For this review, take the finished solid that the model builds, in its own axes (mm). A direction names the side the tool comes from. Round coordinates to 2 decimals unless told otherwise and drop trailing zeros. Write each loop counter-clockwise with the first axis right and the second up, starting at its lowest first coordinate (ties: lowest second). Pieces come first, ordered by that corner, then holes. Notation, with made-up numbers: (54, 35.5) -> (71, 35.5) arc R14 ccw to (71, 59.5) -> close; hole circle Ø1 at (53.5, 36.25). An arc over 180 degrees is marked (long way). Answer in a Markdown table with one row per item. Add a question column.
```python
from build123d import *

# Parameters (mm, degrees)
SKETCH1_R           = 1.75
SKETCH1_W           = 15
SKETCH1_H           = 5.2
SKETCH1_W_2         = 5.2
SKETCH1_H_2         = 30
SKETCH1_H_3         = 15
BOSS_EXTRUDE1_DEPTH = 5


with BuildPart() as part:
    # Sketch1 → Boss-Extrude1 (new body)
    with BuildSketch(Plane(origin=(0, 0, 0), x_dir=(1, 0, 0), z_dir=(0, 1, 0))):
        Polygon((92.514530464, -147.019914311), (92.514530464, 52.980085689), (-80.485469536, 52.980085689), (-130.485469536, 27.980085689), (-213.485469536, 27.980085689), (-213.485469536, -122.019914311), (-130.485469536, -122.019914311), (-80.485469536, -147.019914311), align=None)
        with Locations(Location((62.864530464, -134.489914311, 0), (0, 0, 270))):
            Circle(SKETCH1_R, mode=Mode.SUBTRACT)
        with Locations(Location((41.164530464, -134.489914311, 0), (0, 0, 270))):
            Circle(SKETCH1_R, mode=Mode.SUBTRACT)
        with Locations(Location((62.864530464, -128.139914311, 0), (0, 0, 270))):
            Circle(SKETCH1_R, mode=Mode.SUBTRACT)
        with Locations(Location((41.164530464, -128.139914311, 0), (0, 0, 270))):
            Circle(SKETCH1_R, mode=Mode.SUBTRACT)
        with Locations(Location((62.864530464, -115.439914311, 0), (0, 0, 270))):
            Circle(SKETCH1_R, mode=Mode.SUBTRACT)
        with Locations(Location((41.164530464, -115.439914311, 0), (0, 0, 270))):
            Circle(SKETCH1_R, mode=Mode.SUBTRACT)
        with Locations(Location((62.864530464, -102.739914311, 0), (0, 0, 270))):
            Circle(SKETCH1_R, mode=Mode.SUBTRACT)
        with Locations(Location((41.164530464, -102.739914311, 0), (0, 0, 270))):
            Circle(SKETCH1_R, mode=Mode.SUBTRACT)
        with Locations(Location((41.164530464, 8.700085689, 0), (0, 0, 90))):
            Circle(SKETCH1_R, mode=Mode.SUBTRACT)
        with Locations(Location((41.164530464, 21.400085689, 0), (0, 0, 90))):
            Circle(SKETCH1_R, mode=Mode.SUBTRACT)
        with Locations(Location((41.164530464, 34.100085689, 0), (0, 0, 90))):
            Circle(SKETCH1_R, mode=Mode.SUBTRACT)
        with Locations(Location((41.164530464, 40.450085689, 0), (0, 0, 90))):
            Circle(SKETCH1_R, mode=Mode.SUBTRACT)
        with Locations(Location((62.864530464, 8.700085689, 0), (0, 0, 90))):
            Circle(SKETCH1_R, mode=Mode.SUBTRACT)
        with Locations(Location((62.864530464, 21.400085689, 0), (0, 0, 90))):
            Circle(SKETCH1_R, mode=Mode.SUBTRACT)
        with Locations(Location((62.864530464, 34.100085689, 0), (0, 0, 90))):
            Circle(SKETCH1_R, mode=Mode.SUBTRACT)
        with Locations(Location((62.864530464, 40.450085689, 0), (0, 0, 90))):
            Circle(SKETCH1_R, mode=Mode.SUBTRACT)
        with Locations((75.014530464, 47.380085689)):
            Rectangle(SKETCH1_W, SKETCH1_H, mode=Mode.SUBTRACT)
        with Locations((75.014530464, -141.419914311)):
            Rectangle(SKETCH1_W, SKETCH1_H, mode=Mode.SUBTRACT)
        with Locations((86.914530464, -0.019914311)):
            Rectangle(SKETCH1_W_2, SKETCH1_H_2, mode=Mode.SUBTRACT)
        with Locations((86.914530464, -47.019914311)):
            Rectangle(SKETCH1_W_2, SKETCH1_H_2, mode=Mode.SUBTRACT)
        with Locations((86.914530464, -94.019914311)):
            Rectangle(SKETCH1_W_2, SKETCH1_H_2, mode=Mode.SUBTRACT)
        with Locations((-9.785469536, 47.373767599)):
            Rectangle(SKETCH1_W, SKETCH1_H, mode=Mode.SUBTRACT)
        with Locations((-47.985469536, 47.373767599)):
            Rectangle(SKETCH1_W, SKETCH1_H, mode=Mode.SUBTRACT)
        with Locations((-148.485469536, 22.380085689)):
            Rectangle(SKETCH1_W, SKETCH1_H, mode=Mode.SUBTRACT)
        with Locations((-190.985469536, 22.380085689)):
            Rectangle(SKETCH1_W, SKETCH1_H, mode=Mode.SUBTRACT)
        with Locations((-207.885469536, -3.519914311)):
            Rectangle(SKETCH1_W_2, SKETCH1_H_3, mode=Mode.SUBTRACT)
        with Locations((-207.885469536, -47.019914311)):
            Rectangle(SKETCH1_W_2, SKETCH1_H_2, mode=Mode.SUBTRACT)
        with Locations((-207.885469536, -90.519914311)):
            Rectangle(SKETCH1_W_2, SKETCH1_H_3, mode=Mode.SUBTRACT)
        with Locations((-48.86060515, -141.420106162)):
            Rectangle(SKETCH1_W, SKETCH1_H, mode=Mode.SUBTRACT)
        with Locations((-148.485469536, -116.419914311)):
            Rectangle(SKETCH1_W, SKETCH1_H, mode=Mode.SUBTRACT)
        with Locations((-190.985469536, -116.419914311)):
            Rectangle(SKETCH1_W, SKETCH1_H, mode=Mode.SUBTRACT)
        with Locations((28.414530464, 47.380085689)):
            Rectangle(SKETCH1_W, SKETCH1_H, mode=Mode.SUBTRACT)
        with BuildLine():
            Line((-153.985469536, -47.019914311), (-153.985469536, -44.723390932))
            ThreePointArc((-153.985469536, -44.723390932), (-147.733757287, 12.371069308), (-198.485469536, -14.519914311))
            Line((-198.485469536, -14.519914311), (-198.485469536, -79.519914311))
            ThreePointArc((-198.485469536, -79.519914311), (-147.733757287, -106.41089793), (-153.985469536, -49.31643769))
            Line((-153.985469536, -49.31643769), (-153.985469536, -47.019914311))
        make_face(mode=Mode.SUBTRACT)
        with Locations((28.414530464, -141.419914311)):
            Rectangle(SKETCH1_W, SKETCH1_H, mode=Mode.SUBTRACT)
        with Locations((-9.785469536, -141.413596222)):
            Rectangle(SKETCH1_W, SKETCH1_H, mode=Mode.SUBTRACT)
        Polygon((-110.963133782, 28.573374858), (-113.288285266, 33.223677824), (-126.704693131, 26.515473891), (-124.379541647, 21.865170925), align=None, mode=Mode.SUBTRACT)
        Polygon((-86.455469536, 46.640085689), (-84.130318052, 41.989782723), (-97.546725917, 35.28157879), (-99.871877401, 39.931881756), align=None, mode=Mode.SUBTRACT)
        Polygon((-99.871877401, -133.971710379), (-86.455469536, -140.679914311), (-84.130318052, -136.029611345), (-97.546725917, -129.321407413), align=None, mode=Mode.SUBTRACT)
        Polygon((-124.379541647, -115.904999548), (-110.963133782, -122.61320348), (-113.288285266, -127.263506446), (-126.704693131, -120.555302514), align=None, mode=Mode.SUBTRACT)
    extrude(amount=BOSS_EXTRUDE1_DEPTH)


solid = part.part
```
1. We need section B-B (z = 40.5). Write out the cut boundary in (x, y), plus the area to 3 significant figures.
2. Tool access review of faces 4 (the flat face through (-119.9, 2.46, -29.92)), 5 (the flat face through (-105.835, 2.465, 134.345)): name each direction out of +Z, -Z, +X, -X, +Y, -Y from which nothing blocks a thin tool from reaching the whole face with its end or side.
3. Clearance check with a flat-ended pin moving along its axis: pin 1 Ø4 at (x, z) = (-93.5, 125.5) entering from -Y. State where the tip first meets the part, or that it passes through.
4. We need section A-A (x = 25). Write out the cut boundary in (y, z).
5. We need section C-C (x = -162). Write out the cut boundary in (y, z), plus the area to 3 significant figures.
6. For L1, parallel to Z at x = -49, y = 4.6; L2, parallel to X at y = 3.6, z = 48.5; L3, parallel to X at y = 1.3, z = 10.5, list the stretches that pass through material, from the lowest coordinate up. Write a range as [from, to].
7. We need section D-D (z = 67). Write out the cut boundary in (x, y), plus the area to 3 significant figures.
8. The part is to be moulded in two halves that separate along Z. For faces 1 (the flat face through (-63, 5, 46)), 2 (the flat face through (-105.135, 2.465, -40.655)), 3 (the flat face through (-93.26, 2.46, -43.24)), say which applies: pulls with the +Z half, pulls with the -Z half, needs draft (parallel to the pull), parting line crosses it, or undercut.
Response:
| question | item | result |
|---|---|---|
| 1 | outline | (-213.49, 0) -> (-210.49, 0) -> (-210.49, 5) -> (-213.49, 5) -> close; (-205.29, 0) -> (-198.49, 0) -> (-198.49, 5) -> (-205.29, 5) -> close; (-146.46, 0) -> (84.31, 0) -> (84.31, 5) -> (-146.46, 5) -> close; (89.51, 0) -> (92.51, 0) -> (92.51, 5) -> (89.51, 5) -> close |
| 1 | area | 1,220 mm2 |
| 2 | face 4 | +Y, -Y |
| 2 | face 5 | +Z, -X, +Y, -Y |
| 3 | pin 1 | y = 0 |
| 4 | outline | (0, -52.98) -> (5, -52.98) -> (5, -49.98) -> (0, -49.98) -> close; (0, -44.78) -> (5, -44.78) -> (5, 138.82) -> (0, 138.82) -> close; (0, 144.02) -> (5, 144.02) -> (5, 147.02) -> (0, 147.02) -> close |
| 5 | outline | (0, -27.98) -> (5, -27.98) -> (5, -17.73) -> (0, -17.73) -> close; (0, 111.77) -> (5, 111.77) -> (5, 122.02) -> (0, 122.02) -> close |
| 5 | area | 102 mm2 |
| 6 | L1 | [-52.98, -49.97], [-44.77, 138.82], [144.02, 147.02] |
| 6 | L2 | [-213.49, -210.49], [-205.29, -198.49], [-153.99, 84.31], [89.51, 92.51] |
| 6 | L3 | [-213.49, -210.49], [-205.29, -198.24], [-133.74, 84.31], [89.51, 92.51] |
| 7 | outline | (-213.49, 0) -> (-198.49, 0) -> (-198.49, 5) -> (-213.49, 5) -> close; (-135.99, 0) -> (92.51, 0) -> (92.51, 5) -> (-135.99, 5) -> close |
| 7 | area | 1,220 mm2 |
| 8 | face 1 | needs draft |
| 8 | face 2 | pulls with the -Z half |
| 8 | face 3 | undercut |
